```python
from build123d import *

# Parameters (mm, degrees)
SKETCH_1_R                   = 35.8
EXTRUDE_1_DEPTH              = 47.5
HOLE_WIZARD_M4_1_D           = 3.3
HOLE_WIZARD_M4_1_DEPTH       = 10.1
HOLE_WIZARD_M4_1_CSINK_D     = 4.05
HOLE_WIZARD_M4_1_CSINK_ANGLE = 90
HOLE_WIZARD_M4_1_TIP         = 0.991420021
CHAMFER_1_SIZE               = 1
SKETCH_8_R                   = 30
EXTRUDE_2_DEPTH              = 16
SKETCH_9_R                   = 5.25
EXTRUDE_3_DEPTH              = 20
FILLET_1_R                   = 0.5
HOLE_WIZARD_M5_1_D           = 4.2
HOLE_WIZARD_M5_1_DEPTH       = 12.4
HOLE_WIZARD_M5_1_TIP         = 1.2618073
CUT_EXTRUDE_START            = -12
CUT_EXTRUDE_1_DEPTH          = 12
SKETCH_14_R                  = 1.5
CUT_EXTRUDE_2_DEPTH          = 87.266404315
SKETCH_15_W                  = 12
SKETCH_15_H                  = 24
CUT_EXTRUDE_3_DEPTH          = 5
CHAMFER_2_SIZE               = 1
CHAMFER_2_SIZE2              = 3


with BuildPart() as part:
    # 草图1 → 凸台-拉伸1 (new body)
    with BuildSketch(Plane.XY):
        Circle(SKETCH_1_R)
    extrude(amount=EXTRUDE_1_DEPTH)

    # M4 螺纹孔1
    with Locations(Plane.XY.offset(47.5)):
        with Locations((0, 20), (17.320508076, -10), (-17.320508076, -10)):
            CounterSinkHole(HOLE_WIZARD_M4_1_D / 2, HOLE_WIZARD_M4_1_CSINK_D / 2, depth=HOLE_WIZARD_M4_1_DEPTH, counter_sink_angle=HOLE_WIZARD_M4_1_CSINK_ANGLE)
            with Locations((0, 0, -(HOLE_WIZARD_M4_1_DEPTH + HOLE_WIZARD_M4_1_TIP / 2))):  # 118° drill point
                Cone(0, HOLE_WIZARD_M4_1_D / 2, HOLE_WIZARD_M4_1_TIP, mode=Mode.SUBTRACT)

    # 倒角1
    chamfer_1_edges = [part.edges().sort_by_distance(p)[0] for p in [
        (-35.8, 0, 0),
        (-35.8, 0, 47.5),
    ]]
    chamfer(chamfer_1_edges, length=CHAMFER_1_SIZE)

    # 草图8 → 凸台-拉伸2 (add)
    with BuildSketch(Plane(origin=(0, 0, 0), x_dir=(-1, 0, 0), z_dir=(0, 0, -1))):
        with Locations(Location((0, 0, 0), (0, 0, 180))):
            Circle(SKETCH_8_R)
    extrude(amount=EXTRUDE_2_DEPTH)

    # 草图9 → 凸台-拉伸3 (add)
    with BuildSketch(Plane.XY.offset(47.5)):
        Circle(SKETCH_9_R)
    extrude(amount=EXTRUDE_3_DEPTH)

    # 圆角1
    fillet_1_edges = [part.edges().sort_by_distance(p)[0] for p in [
        (-5.25, 0, 67.5),
    ]]
    fillet(fillet_1_edges, radius=FILLET_1_R)

    # M5 螺纹孔1
    with Locations(Plane.XY.offset(67.5)):
        with Locations((0, 0)):
            Hole(HOLE_WIZARD_M5_1_D / 2, depth=HOLE_WIZARD_M5_1_DEPTH)
            with Locations((0, 0, -(HOLE_WIZARD_M5_1_DEPTH + HOLE_WIZARD_M5_1_TIP / 2))):  # 118° drill point
                Cone(0, HOLE_WIZARD_M5_1_D / 2, HOLE_WIZARD_M5_1_TIP, mode=Mode.SUBTRACT)

    # 草图13 → 切除-拉伸1 (cut)
    with BuildSketch(Plane.XY.offset(67.5).offset(CUT_EXTRUDE_START)):
        with BuildLine():
            Line((-3.082207001, 4.25), (3.082207001, 4.25))
            ThreePointArc((3.082207001, 4.25), (0, 5.25), (-3.082207001, 4.25))
        make_face()
    extrude(amount=CUT_EXTRUDE_1_DEPTH, mode=Mode.SUBTRACT)

    # 草图14 → 切除-拉伸2 (cut, through all)
    with BuildSketch(Plane(origin=(0, 4.25, 0), x_dir=(1, 0, 0), z_dir=(0, 1, 0))):
        with Locations(Location((0, -64.5, 0), (0, 0, 270))):
            Circle(SKETCH_14_R)
    extrude(amount=-CUT_EXTRUDE_2_DEPTH, mode=Mode.SUBTRACT)

    # 草图15 → 切除-拉伸3 (cut)
    with BuildSketch(Plane(origin=(30, 0, 0), x_dir=(0, 0, -1), z_dir=(1, 0, 0))):
        with Locations((6, 0)):
            Rectangle(SKETCH_15_W, SKETCH_15_H)
    extrude(amount=-CUT_EXTRUDE_3_DEPTH, mode=Mode.SUBTRACT)

    # 倒角2
    chamfer_2_edges = [part.edges().sort_by_distance(p)[0] for p in [
        (-30, 0, -16),
    ]]
    chamfer_2_side = [part.faces().sort_by_distance(p)[0] for p in [
        (-30, 0, -8),
    ]]
    chamfer(chamfer_2_edges, length=CHAMFER_2_SIZE, length2=CHAMFER_2_SIZE2, reference=chamfer_2_side[0])


solid = part.part
```
Geometry: final body of the model. Coordinates: model frame, mm. A direction names the side the tool comes from. Round coordinates to 2 decimals unless told otherwise and drop trailing zeros. Loops run counter-clockwise (first coordinate to the right, second up) from the corner with the lowest first, then second, coordinate; pieces in that order, holes last. Notation, with made-up numbers: (69, 59.25) -> (121, 59.25) arc R17 ccw to (121, 77.25) -> close; hole circle Ø11 at (59.5, -24.75). An arc over 180 degrees is marked (long way). Use one line per item in the form item = value. Start each with the question number.
1) First-contact query: P1, Ø5, axis at x = 0.5, z = 63, coming from the +Y side; P2, Ø3.5, axis at x = 0, z = 64.5, coming from the -Y side; P3, Ø8, axis at x = -22, y = -18, coming from the +Z side. Flat tips, straight axial feed; report the tip coordinate or a pass-through.
2) Section B-B on z = 52.5. Output: boundary loops of the cut face in (x, y).
3) Draft query along X for faces 4 (the cylindrical face through (-1.138, -5.125, 57.114)), 5 (the flat face through (1, -2.2, 67.5)), 6 (the cylindrical face through (15.796, -10.632, 42.194)). Return one class per face: released by +X, released by -X, zero draft, split by the parting line, or undercut.
4) Section C-C on z = -9. Output: boundary loops of the cut face in (x, y), then the cut area to 3 significant figures.
5) Access query for faces 1 (the cylindrical face through (2.1, 0.09, 61.21)), 2 (the flat face through (0, 4.25, 61)), 3 (the flat face through (25, 0, -6)). Directions: +Z, -Z, +X, -X, +Y, -Y. A direction counts if a zero-diameter tool reaches every point of the face in a straight line with its end or side. Return the directions, or none.
6) Section D-D on z = 25. Output: boundary loops of the cut face in (x, y).
7) Line query: L1, parallel to Z at x = 0, y = -3.15; L2, parallel to X at y = -10, z = 44 (1 decimal); L3, parallel to X at y = 0, z = 59. Output: solid intervals per line, ascending.
8) Section A-A on z = 64.5. Output: boundary loops of the cut face in (x, y), then the cut area to 3 significant figures.
Response:
q1.P1 = 4.25
q1.P2 = -5.25
q1.P3 = 47.5
q2.outline = circle Ø10.5 at (0, 0)
q3.face_4 = split by the parting line
q3.face_5 = zero draft
q3.face_6 = undercut
q4.outline = (25, -12) -> (25, 12) -> (27.5, 12) arc R30 ccw (long way) to (27.5, -12) -> close
q4.area = 2,730 mm^2
q5.face_1 = +Z
q5.face_2 = +Z, +X, -X, +Y
q5.face_3 = +X
q6.outline = circle Ø71.6 at (0, 0)
q7.L1 = -16 to 63, 66 to 67.5
q7.L2 = -34.4 to -19, -15.7 to 15.7, 19 to 34.4
q7.L3 = -5.25 to -2.1, 2.1 to 5.25
q8.outline = (-3.08, 4.25) arc R5.25 ccw to (-1.5, -5.03) -> (-1.5, -1.47) arc R2.1 cw to (-1.5, 1.47) -> (-1.5, 4.25) -> close; (1.5, -5.03) arc R5.25 ccw to (3.08, 4.25) -> (1.5, 4.25) -> (1.5, 1.47) arc R2.1 cw to (1.5, -1.47) -> close
q8.area = 51.7 mm^2
